Work out the finished part from the listing and answer in its coordinate system (mm). A direction names the side the tool comes from. Round coordinates to 2 decimals unless told otherwise and drop trailing zeros. Write each loop counter-clockwise with the first axis right and the second up, starting at its lowest first coordinate (ties: lowest second). Pieces come first, ordered by that corner, then holes. Notation, with made-up numbers: (48, 47.25) - (84, 47.25) arc R16 cw to (84, 60.25) - close; hole circle Ø3 at (77.5, 68). An arc over 180 degrees is marked (long way). Answer as a JSON object with one key per item and string values.
```python
from build123d import *

# Parameters (mm, degrees)
F1_DEPTH = 127
F2_SIZE  = 5.08
F4_D     = 2.54
F5_R     = 6.35
F6_SIZE  = 2.54


with BuildPart() as f1:
    # F0 (on Right) → F1 (new body)
    with BuildSketch(Plane.YZ):
        Polygon((0, 2.54), (0, 0), (33.02, 0), (33.02, 41.91), (53.34, 41.91), (53.34, 45.72), (27.94, 45.72), (27.94, 2.54), align=None)
    extrude(amount=-F1_DEPTH)

    # F2
    f2_edges = [f1.edges().sort_by_distance(p)[0] for p in [
        (0, 0, 1.27),
        (-127, 0, 1.27),
    ]]
    chamfer(f2_edges, length=F2_SIZE)

    # F4 (through all)
    with Locations(Plane.XY.offset(45.72)):
        with Locations((-120.65, 40.64), (-82.55, 40.64), (-44.45, 40.64), (-6.35, 40.64)):
            Hole(F4_D / 2)

    # F5
    f5_edges = [f1.edges().sort_by_distance(p)[0] for p in [
        (0, 53.34, 43.815),
        (-127, 53.34, 43.815),
    ]]
    fillet(f5_edges, radius=F5_R)

    # F6
    f6_edges = [f1.edges().sort_by_distance(p)[0] for p in [
        (-63.5, 33.02, 0),
    ]]
    chamfer(f6_edges, length=F6_SIZE)


solid = f1.part
```
Item 1: A cutting plane is placed at C-C (z = 36.5). Write down the section's boundary in (x, y), and give its area (3 significant figures).
Results found:
{"outline": "(-127, 27.94) - (0, 27.94) - (0, 33.02) - (-127, 33.02) - close", "area": "645 mm²"}
Item 2: Determine the mould class of faces 4 (the cylindrical face through (-6.2, 41.9, 43.8)), 5 (the flat face through (-124.5, 2.58, 1.29)), 6 (the flat face through (-63, 43, 41.91)) for opening direction Y: pulls with the +Y half, pulls with the -Y half, needs draft (parallel to the pull), parting line crosses it, or undercut.
Results found:
{"face 4": "undercut", "face 5": "pulls with the -Y half", "face 6": "needs draft"}
Item 3: For faces 1 (the flat face through (-63, 33.02, 22)), 2 (the cylindrical face through (-44.3, 41.9, 43.8)), 3 (the flat face through (-63, 14, 2.54)), determine the directions among +Z, -Z, +X, -X, +Y, -Y from which every point of the face is accessible in a straight line to the end or side of a thin tool.
Results found:
{"face 1": "-Z, +X, -X, +Y", "face 2": "+Z, -Z", "face 3": "+Z, +X, -X, -Y"}
Item 4: A cutting plane is placed at B-B (y = 40.64). Write down the section's boundary in (x, z).
Results found:
{"outline": "(-127, 41.91) - (-121.92, 41.91) - (-121.92, 45.72) - (-127, 45.72) - close; (-119.38, 41.91) - (-83.82, 41.91) - (-83.82, 45.72) - (-119.38, 45.72) - close; (-81.28, 41.91) - (-45.72, 41.91) - (-45.72, 45.72) - (-81.28, 45.72) - close; (-43.18, 41.91) - (-7.62, 41.91) - (-7.62, 45.72) - (-43.18, 45.72) - close; (-5.08, 41.91) - (0, 41.91) - (0, 45.72) - (-5.08, 45.72) - close"}
Item 5: A cutting plane is placed at A-A (x = -82.55). Write down the section's boundary in (y, z), and give its area (3 significant figures).
Results found:
{"outline": "(0, 0) - (30.48, 0) - (33.02, 2.54) - (33.02, 41.91) - (39.37, 41.91) - (39.37, 45.72) - (27.94, 45.72) - (27.94, 2.54) - (0, 2.54) - close; (41.91, 41.91) - (53.34, 41.91) - (53.34, 45.72) - (41.91, 45.72) - close", "area": "368 mm²"}
Item 6: Consider line 1 along Y through (x, z) = (-44.45, 42.7); line 2 along X through (y, z) = (40, 44); line 3 along Y through (x, z) = (-67, 28.5). Determine where each line is inside the solid, lowest interval first.
Results found:
{"line 1": "27.94 to 39.37, 41.91 to 53.34", "line 2": "-127 to -121.75, -119.55 to -83.65, -81.45 to -45.55, -43.35 to -7.45, -5.25 to 0", "line 3": "27.94 to 33.02"}
Item 7: Each of these flat-tipped pins is pushed along its axis until it touches: P1, Ø12, axis at x = -39, z = 11.5, coming from the -Y side; P2, Ø3, axis at x = -6.35, y = 40.64, coming from the -Z side; P3, Ø3, axis at x = -79.5, y = 14, coming from the +Z side. Where does it stop, or does it pass through?
Results found:
{"P1": "y = 27.94", "P2": "z = 41.91", "P3": "z = 2.54"}
Item 8: A cutting plane is placed at D-D (y = 21). Write down the section's boundary in (x, z), and give its area (3 significant figures).
Results found:
{"outline": "(-127, 0) - (0, 0) - (0, 2.54) - (-127, 2.54) - close", "area": "323 mm²"}
